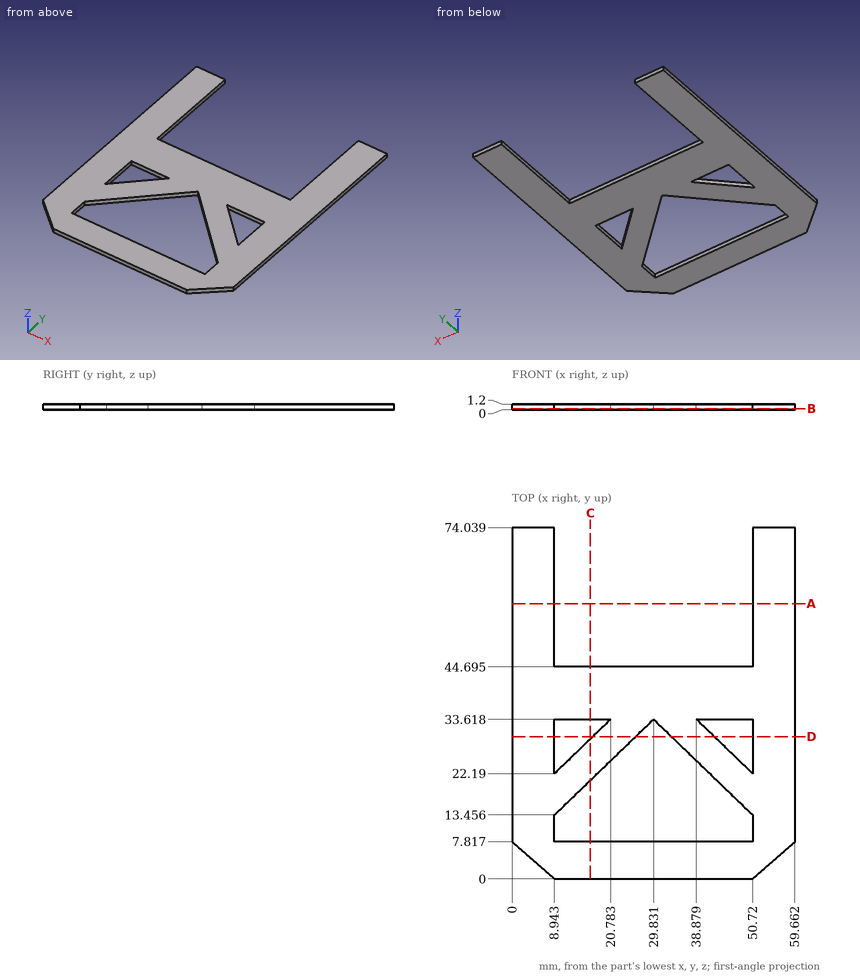
Drawing for the job (mm, zero at the part's lowest x, y, z). Round coordinates to 2 decimals unless told otherwise and drop trailing zeros. Loops run counter-clockwise (first coordinate to the right, second up) from the corner with the lowest first, then second, coordinate; pieces in that order, holes last. Notation, with made-up numbers: (44.5, 61) -> (95.5, 61) arc R12 ccw to (95.5, 80) -> close; hole circle Ø10 at (54, -24.5). An arc over 180 degrees is marked (long way). Answer as CSV lines item,"result". Start each with the question number.
1) Probe line 1 along X through (y, z) = (32, 0.2) (1 decimal); line 2 along X through (y, z) = (31, 0.45) (1 decimal); line 3 along X through (y, z) = (56, 0.5). List the from-to ranges inside material, lowest first.
2) Slice it at D-D (y = 30). List the corners of the cut face in (x, z) (1 decimal).
3) Slice it at B-B (z = 0.25). List the corners of the cut face in (x, y) (1 decimal).
4) Slice it at A-A (y = 58). List the corners of the cut face in (x, z).
5) Pin check, flat tip, straight feed: P1, Ø12, axis at x = 51, y = 37.5, coming from the -Z side. Stop position of the tip, or through.
6) Slice it at C-C (x = 16.5). State how many separate pieces and enclosed holes the cut face has.
Filled in:
1,line 1,"x = 0 to 8.9, 19.1 to 28.2, 31.5 to 40.6, 50.7 to 59.7"
1,line 2,"x = 0 to 8.9, 18.1 to 27.1, 32.5 to 41.6, 50.7 to 59.7"
1,line 3,"x = 0 to 8.94, 50.72 to 59.66"
2,outline,"(0, 0) -> (8.9, 0) -> (8.9, 1.2) -> (0, 1.2) -> close; (17, 0) -> (26.1, 0) -> (26.1, 1.2) -> (17, 1.2) -> close; (33.6, 0) -> (42.6, 0) -> (42.6, 1.2) -> (33.6, 1.2) -> close; (50.7, 0) -> (59.7, 0) -> (59.7, 1.2) -> (50.7, 1.2) -> close"
3,outline,"(0, 7.8) -> (8.9, 0) -> (50.7, 0) -> (59.7, 7.8) -> (59.7, 74) -> (50.7, 74) -> (50.7, 44.7) -> (8.9, 44.7) -> (8.9, 74) -> (0, 74) -> close; hole (8.9, 7.8) -> (50.7, 7.8) -> (50.7, 13.5) -> (29.8, 33.6) -> (8.9, 13.5) -> close; hole (8.9, 22.2) -> (20.8, 33.6) -> (8.9, 33.6) -> close; hole (38.9, 33.6) -> (50.7, 22.2) -> (50.7, 33.6) -> close"
4,outline,"(0, 0) -> (8.94, 0) -> (8.94, 1.2) -> (0, 1.2) -> close; (50.72, 0) -> (59.66, 0) -> (59.66, 1.2) -> (50.72, 1.2) -> close"
5,P1,"stops at z = 0"
6,separate pieces,"3"
6,enclosed holes,"0"
